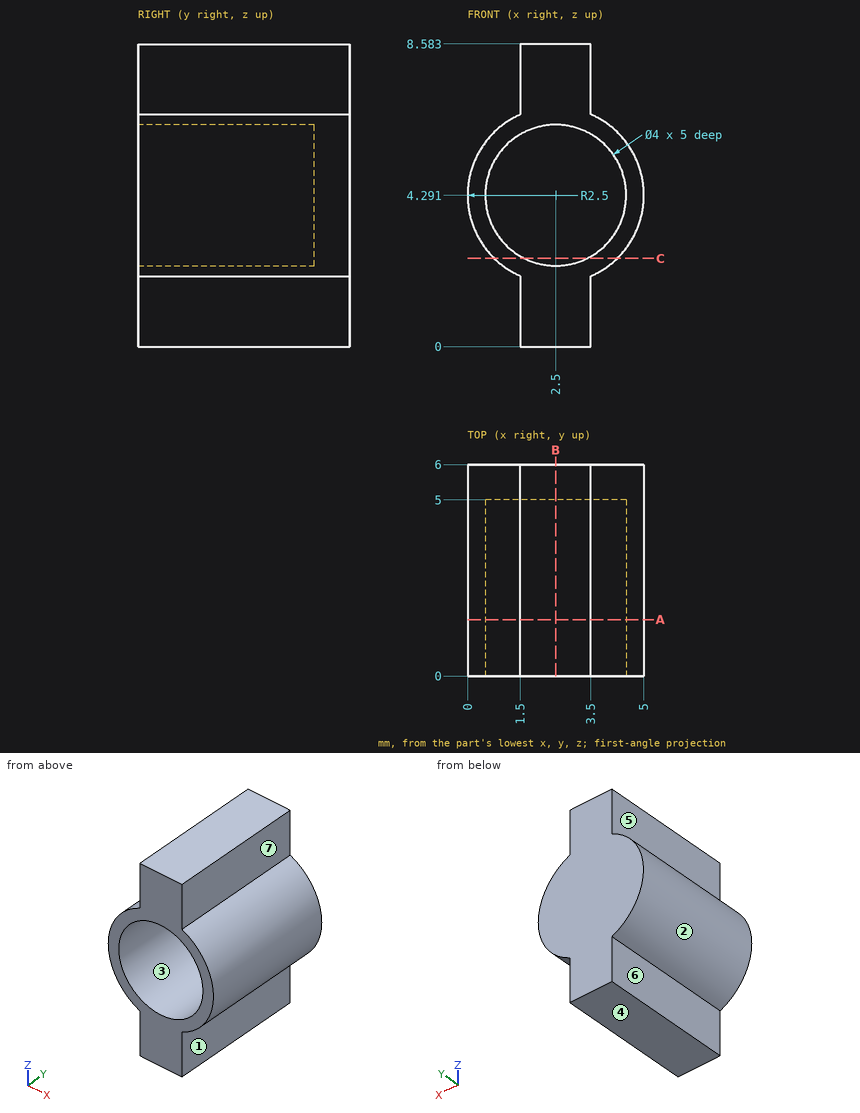
Study the drawing (mm; zero at the part's minimum x, y, z) and answer. A direction names the side the tool comes from. Round coordinates to 2 decimals unless told otherwise and drop trailing zeros. Write each loop counter-clockwise with the first axis right and the second up, starting at its lowest first coordinate (ties: lowest second). Pieces come first, ordered by that corner, then holes.
1) Given pin 1 Ø1 at (y, z) = (1.5, 6.5) entering from +X (1 decimal); pin 2 Ø1.5 at (x, z) = (2, 5) entering from -Y; pin 3 Ø0.6 at (y, z) = (2.5, 0.5) entering from -X, each flat-ended and moving along its own axis, determine where each tip first touches the part or whether it passes through.
2) The mould has two halves that part along X. Classify the marked faces 1, 2 and 3: pulls with the +X half, pulls with the -X half, needs draft (parallel to the pull), parting line crosses it, or undercut.
3) A cutting plane is placed at A-A (y = 1.6). Give the vertices of the cut face in (x, z), plus the area to 3 significant figures.
4) A tool of negligible diameter and unlimited length cuts with its end or side. For the marked faces 4, 5, 6 and 7, from which of +Z, -Z, +X, -X, +Y, -Y can it reach the whole face along a straight path? Write none if from no direction.
5) A cutting plane is placed at B-B (x = 2.5). Give the vertices of the cut face in (y, z).
6) Straight lines are drawn through the part: line 1 (X direction, y = 4.5, z = 4.25); line 2 (X direction, y = 2.2, z = 7.75); line 3 (Y direction, x = 3.35, z = 3.25). For each, find the intervals that lie inside material, in ascending order.
7) A cutting plane is placed at C-C (z = 2.5). Give the vertices of the cut face in (x, y).
Completed:
1. pin 1: stops at x = 4.3
1. pin 2: stops at y = 5
1. pin 3: stops at x = 1.5
2. face 1: pulls with the +X half
2. face 2: pulls with the -X half
2. face 3: undercut
3. outline: (1.5, 0) - (3.5, 0) - (3.5, 2) arc R2.5 ccw to (3.5, 6.58) - (3.5, 8.58) - (1.5, 8.58) - (1.5, 6.58) arc R2.5 ccw to (1.5, 2) - close; hole circle Ø4 at (2.5, 4.29)
3. area: 14.5 mm2
4. face 4: -Z, +X, -X, +Y, -Y
4. face 5: +Z, -X, +Y, -Y
4. face 6: -Z, -X, +Y, -Y
4. face 7: +Z, +X, +Y, -Y
5. outline: (0, 0) - (6, 0) - (6, 8.58) - (0, 8.58) - (0, 6.29) - (5, 6.29) - (5, 2.29) - (0, 2.29) - close
6. line 1: x = 0 to 0.5, 4.5 to 5
6. line 2: x = 1.5 to 3.5
6. line 3: y = 5 to 6
7. outline: (0.76, 0) - (1.61, 0) - (1.61, 5) - (3.39, 5) - (3.39, 0) - (4.24, 0) - (4.24, 6) - (0.76, 6) - close
